from build123d import *

# Parameters (mm, degrees)
F1_DEPTH = 1.5875
F3_DEPTH = 19.05


with BuildPart() as f1:
    # F0 (on Top) → F1 (new body)
    with BuildSketch(Plane.XY):
        with BuildLine():
            Line((40.410568, 15.044903), (27.710568, 15.044903))
            Line((27.710568, 15.044903), (27.710568, -23.055097))
            Line((27.710568, -23.055097), (40.410568, -23.055097))
            ThreePointArc((40.410568, -23.055097), (44.900696, -21.195225), (46.760568, -16.705097))
            Line((46.760568, -16.705097), (46.760568, 8.694903))
            ThreePointArc((46.760568, 8.694903), (44.900696, 13.185031), (40.410568, 15.044903))
        make_face()
    extrude(amount=F1_DEPTH)

    # F2 (on face) → F3 (join)
    with BuildSketch(Plane.XY.offset(1.5875)):
        with BuildLine():
            Line((27.710568, 15.044903), (27.710568, 13.457403))
            Line((27.710568, 13.457403), (38.823068, 13.457403))
            ThreePointArc((38.823068, 13.457403), (43.313196, 11.597531), (45.173068, 7.107403))
            Line((45.173068, 7.107403), (45.173068, -15.117597))
            ThreePointArc((45.173068, -15.117597), (43.313196, -19.607725), (38.823068, -21.467597))
            Line((38.823068, -21.467597), (27.710568, -21.467597))
            Line((27.710568, -21.467597), (27.710568, -23.055097))
            Line((27.710568, -23.055097), (40.410568, -23.055097))
            ThreePointArc((40.410568, -23.055097), (44.900696, -21.195225), (46.760568, -16.705097))
            Line((46.760568, -16.705097), (46.760568, 8.694903))
            ThreePointArc((46.760568, 8.694903), (44.900696, 13.185031), (40.410568, 15.044903))
            Line((40.410568, 15.044903), (27.710568, 15.044903))
        make_face()
    extrude(amount=-F3_DEPTH)


solid = f1.part
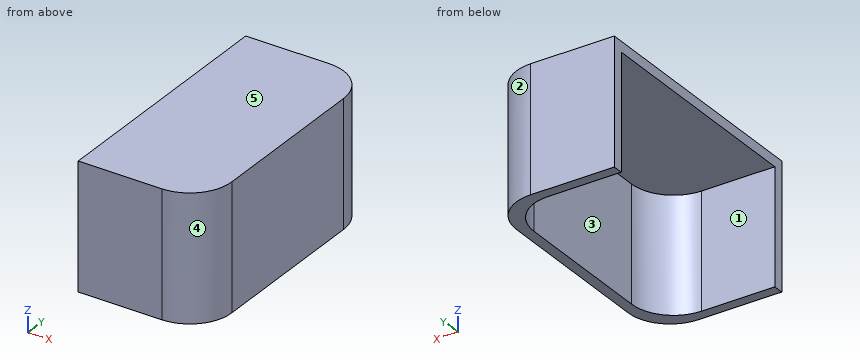
The model under review builds one solid part; all positions refer to its coordinate system, in mm. Face numbers are marked on the shaded views. A direction names the side the tool comes from. Round coordinates to 2 decimals unless told otherwise and drop trailing zeros. Write each loop counter-clockwise with the first axis right and the second up, starting at its lowest first coordinate (ties: lowest second). Pieces come first, ordered by that corner, then holes. Notation, with made-up numbers: M -25.75,26.25 L -8.75,26.25 A29 cw -8.75,56.25 Z; hole C 86.5,84.5 d3. An arc over 180 degrees is marked long. Use a Markdown table: item, result. Add a question column.
Q1. The part is to be moulded in two halves that separate along Y. For the marked faces 3, 4 and 5, say which applies: pulls with the +Y half, pulls with the -Y half, needs draft (parallel to the pull), parting line crosses it, or undercut.
Q2. Machinability: for the marked faces 1 and 2, which of the approach directions +Z, -Z, +X, -X, +Y, -Y give a long, thin tool a straight path to every point of the face, cutting with its end or side? Answer none if there is none.
Q3. We need section B-B, the plane x = 34.5. State the section outline as (y, z) points.
Q4. To check wall thickness, follow line 1 (Y direction, x = 38.25, z = -13.75); line 2 (Z direction, x = 30.75, y = -15); line 3 (X direction, y = -1.5, z = -14.75). State the ranges of each line that lie inside material, in increasing order.
Q5. Insertion check: pin 1 (1 mm diameter, centred on y = -5, z = -10.5, fed in from -X). The pin has a flat end and moves straight along its axis. Give the tip position at first contact, or say it passes through.
Q6. We need section A-A, the plane z = -4.75. State the section outline as (x, y) points, plus the area to 3 significant figures.
Q7. We need section C-C, the plane y = 1. State the section outline as (x, z) points, plus the area to 3 significant figures.
Q8. We need section D-D, the plane y = 11. State the section outline as (x, z) points.
Findings below:
| question | item | result |
|---|---|---|
| 1 | face 3 | undercut |
| 1 | face 4 | pulls with the -Y half |
| 1 | face 5 | needs draft |
| 2 | face 1 | -Z, -X |
| 2 | face 2 | +Z, -Z, +X, +Y |
| 3 | outline | M -23.06,-17.46 L -21.47,-17.46 L -21.47,0 L 13.46,0 L 13.46,-17.46 L 15.04,-17.46 L 15.04,1.59 L -23.06,1.59 Z |
| 4 | line 1 | y = -23.06 to -21.47, 13.46 to 15.04 |
| 4 | line 2 | z = 0 to 1.59 |
| 4 | line 3 | x = 45.17 to 46.76 |
| 5 | pin 1 | stops at x = 45.17 |
| 6 | outline | M 27.71,-23.06 L 40.41,-23.06 A6.35 ccw 46.76,-16.71 L 46.76,8.69 A6.35 ccw 40.41,15.04 L 27.71,15.04 L 27.71,13.46 L 38.82,13.46 A6.35 cw 45.17,7.11 L 45.17,-15.12 A6.35 cw 38.82,-21.47 L 27.71,-21.47 Z |
| 6 | area | 116 mm² |
| 7 | outline | M 27.71,0 L 45.17,0 L 45.17,-17.46 L 46.76,-17.46 L 46.76,1.59 L 27.71,1.59 Z |
| 7 | area | 58.0 mm² |
| 8 | outline | M 27.71,0 L 43.84,0 L 43.84,-17.46 L 46.33,-17.46 L 46.33,1.59 L 27.71,1.59 Z |
